```python
from build123d import *

# Parameters (mm, degrees)
CUT_EXTRUDE_1_DEPTH = 13.4
SKETCH_4_R          = 2.1
CUT_EXTRUDE_2_DEPTH = 13.4


with BuildPart() as part:
    # 草图2 → 旋转1 (revolve)
    with BuildSketch(Plane(origin=(0, 0, 0), x_dir=(1, 0, 0), z_dir=(0, 1, 0))):
        Polygon((-21.742218247, 43.984257603), (-18.742218247, 43.984257603), (-18.742218247, 23.034257603), (-11.742218247, 18.979304476), (-11.742218247, -20.515742397), (-19.242218247, -20.515742397), (-19.242218247, 6.984257603), (-20.242218247, 6.984257603), (-20.242218247, 7.984257603), (-21.742218247, 7.984257603), (-21.742218247, 11.984257603), (-38.612218247, 11.984257603), (-38.612218247, 15.984257603), (-21.742218247, 15.984257603), align=None)
    revolve(axis=Axis((-11.742218247, 0, -18.979304476), (0, 0, 1)))

    # 草图3 → 切除-拉伸1 (cut)
    with BuildSketch(Plane.XY.offset(20.515742397)):
        with BuildLine():
            Line((-11.742218247, 4), (-14.742218247, 4))
            ThreePointArc((-14.742218247, 4), (-11.742218247, -5), (-8.742218247, 4))
            Line((-8.742218247, 4), (-11.742218247, 4))
        make_face()
    extrude(amount=-CUT_EXTRUDE_1_DEPTH, mode=Mode.SUBTRACT)

    # 草图4 → 切除-拉伸2 (cut)
    with BuildSketch(Plane.XY.offset(-11.984257603)):
        with Locations((-0.492218247, -18.86)):
            Circle(SKETCH_4_R)
        with Locations((10.757781753, 0)):
            Circle(SKETCH_4_R)
        with Locations((-22.992218247, -18.86)):
            Circle(SKETCH_4_R)
        with Locations((-34.242218247, 0)):
            Circle(SKETCH_4_R)
        with Locations((-22.992218247, 18.86)):
            Circle(SKETCH_4_R)
        with Locations((-0.492218247, 18.86)):
            Circle(SKETCH_4_R)
    extrude(amount=-CUT_EXTRUDE_2_DEPTH, mode=Mode.SUBTRACT)


solid = part.part
```
Design review of the part built by this model. Coordinates are the model's own, in mm. A direction names the side the tool comes from. Coordinates: 2 decimals unless noted, no trailing zeros. Order: outer loops, then holes, each group sorted by start corner. A loop starts at its lowest first (then second) coordinate and runs counter-clockwise, first axis right, second up.
1) For faces 1 (the flat face through (-14.8, 8.1, -7.984)), 2 (the flat face through (-12, 5, 20.516)), 3 (the cylindrical face through (-9.57, 9.76, -30.18)), list the 3-axis set-ups (+Z, -Z, +X, -X, +Y, -Y) from which the entire face can be reached by the end or side of a thin tool; tool diameter is ignored.
2) Clearance check with flat-ended pins moving along their axes: pin 1 (4 mm diameter, centred on x = -26.5, y = 4.5, fed in from +Z); pin 2 (12 mm diameter, centred on y = 17, z = -11.5, fed in from +X); pin 3 (2 mm diameter, centred on x = 4.5, y = -6, fed in from -Z); pin 4 (13 mm diameter, centred on x = -11.74, y = 0, fed in from +Z). State where each tip first meets the part, or that it passes through.
3) Take a section at B-B, the plane y = 18.86. Give the boundary of the cut face in (x, z), and give its area (3 significant figures).
4) Mouldability with a two-part tool opening along Y and no side actions: class faces 4 (the cylindrical face through (-4.25, -0.33, 6.57)), 5 (the cylindrical face through (8.66, 0.09, -13.96)), 6 (the flat face through (0, 0, -11.984)), 7 (the cylindrical face through (-4.75, -0.31, -33.36)) as +Y half, -Y half, draft (parallel to the pull), parting line (faces both ways), or undercut.
5) Take a section at C-C, the plane z = -27. Give the boundary of the cut face in (x, y), and give its area (3 significant figures).
6) Wall thickness on line 1 along X through (y, z) = (-18, -13); line 2 along Z through (x, y) = (11.5, -4.5); line 3 along X through (y, z) = (0, 17.5): over which ranges is each line inside the solid? List them lowest first.
7) Take a section at D-D, the plane z = 0. Give the boundary of the cut face in (x, y), and give its area (3 significant figures).
8) Take a section at A-A, the plane z = -13. Give the boundary of the cut face in (x, y).
Returned:
1. face 1: +Z
1. face 2: +Z, +X, -X, +Y, -Y
1. face 3: -Z
2. pin 1: stops at z = -11.98
2. pin 2: stops at x = 12.76
2. pin 3: stops at z = -15.98
2. pin 4: stops at z = 20.52
3. outline: (-30.88, -15.98) - (-25.09, -15.98) - (-25.09, -11.98) - (-30.88, -11.98) - close; (-20.89, -15.98) - (-2.59, -15.98) - (-2.59, -11.98) - (-20.89, -11.98) - close; (1.61, -15.98) - (7.4, -15.98) - (7.4, -11.98) - (1.61, -11.98) - close
3. area: 120 mm2
4. face 4: parting line
4. face 5: undercut
4. face 6: draft
4. face 7: undercut
5. outline: circle Ø20 at (-11.74, 0); hole circle Ø14 at (-11.74, 0)
5. area: 160 mm2
6. line 1: x = -31.69 to -24.91, -21.08 to -2.41, 1.42 to 8.21
6. line 2: z = -15.98 to -11.98
6. line 3: x = -19.24 to -16.74, -6.74 to -4.24
7. outline: circle Ø15 at (-11.74, 0)
7. area: 177 mm2
8. outline: circle Ø53.74 at (-11.74, 0); hole circle Ø4.2 at (-34.24, 0); hole circle Ø4.2 at (-22.99, -18.86); hole circle Ø4.2 at (-22.99, 18.86); hole circle Ø4.2 at (-0.49, -18.86); hole circle Ø4.2 at (-0.49, 18.86); hole circle Ø4.2 at (10.76, 0)
